Input: part model. Units: mm. Frame: model coordinates. Face numbers are marked on the shaded views. A direction names the side the tool comes from. Coordinates: 2 decimals unless noted, no trailing zeros. Order: outer loops, then holes, each group sorted by start corner. A loop starts at its lowest first (then second) coordinate and runs counter-clockwise, first axis right, second up. Notation, with made-up numbers: (22.5, 44) - (45.5, 44) arc R14 ccw to (45.5, 50) - close; hole circle Ø3 at (10.25, 6). An arc over 180 degrees is marked (long way). Answer as CSV lines item,"result". Start each with the question number.
Item 1: Material intervals for line 1 along Y through (x, z) = (-15, 31.4); line 2 along X through (y, z) = (-12.5, 31.6); line 3 along Z through (x, y) = (48.5, -15.5), sorted ascending.
Item 2: First-contact query: pin 1 (0.6 mm diameter, centred on x = -15, z = 29, fed in from +Y); pin 2 (4 mm diameter, centred on x = 20.5, z = 23.5, fed in from +Y); pin 3 (6.5 mm diameter, centred on x = -15, y = -0.5, fed in from -Z). Flat tips, straight axial feed; report the tip coordinate or a pass-through.
Item 3: Section C-C (z = 24.25). Output: boundary loops of the cut face in (x, y).
Item 4: Access query for the marked faces 1, 2 and 3. Directions: +Z, -Z, +X, -X, +Y, -Y. A direction counts if a zero-diameter tool reaches every point of the face in a straight line with its end or side. Return the directions, or none.
Item 5: Section B-B (x = -15). Output: boundary loops of the cut face in (y, z), and give its area (3 significant figures).
Item 6: Section A-A (y = 15.5). Output: boundary loops of the cut face in (x, z), and give its area (4 significant figures).
Item 7: Draft query along X for the marked faces 4, 5 and 6. Return one class per face: +X half, -X half, draft (parallel to the pull), parting line (faces both ways), or undercut.
Item 8: Section D-D (x = 13). Output: boundary loops of the cut face in (y, z).
from build123d import *

# Parameters (mm, degrees)
CYLINDER026_R     = 3.15
CYLINDER026_DEPTH = 10
CYLINDER027_R     = 3.15
CYLINDER027_DEPTH = 10
CYLINDER028_R     = 1.65
CYLINDER028_DEPTH = 83
CYLINDER029_R     = 1.65
CYLINDER029_DEPTH = 83
BOX022_W          = 50.5
BOX022_H          = 8
BOX022_DEPTH      = 9
CHAMFER026_SIZE   = 7
CYLINDER025_R     = 17
CYLINDER025_DEPTH = 83
BOX021_W          = 5
BOX021_H          = 57
BOX021_DEPTH      = 10
CHAMFER027_SIZE   = 1
BOX024_W          = 8
BOX024_H          = 16
BOX024_DEPTH      = 2
BOX036_W          = 28
BOX036_H          = 14
BOX036_DEPTH      = 10
BOX023_W          = 77.5
BOX023_H          = 57
BOX023_DEPTH      = 5
FILLET002_R       = 3


with BuildPart() as cylinder012:
    # Cylinder026 → Cylinder026 (new body)
    with BuildSketch(Plane(origin=(-15, 11.5, 26), x_dir=(1, 0, 0), z_dir=(0, 0, 1))):
        Circle(CYLINDER026_R)
    extrude(amount=CYLINDER026_DEPTH)


with BuildPart() as fusion006002011004053036004001028003008:
    # Cylinder027 → Cylinder027 (new body)
    with BuildSketch(Plane(origin=(-15, -12.5, 26), x_dir=(1, 0, 0), z_dir=(0, 0, 1))):
        Circle(CYLINDER027_R)
    extrude(amount=CYLINDER027_DEPTH)

    # Fusion006002011004053036004001028003008: union Cylinder012
    add(cylinder012.part)


with BuildPart() as obj1:
    # Cylinder028 → Cylinder028 (new body)
    with BuildSketch(Plane(origin=(25.5, -15.5, 24), x_dir=(0, 0, -1), z_dir=(1, 0, 0))):
        Circle(CYLINDER028_R)
    extrude(amount=CYLINDER028_DEPTH)


with BuildPart() as fusion006002011004053036004001024:
    # Cylinder029 → Cylinder029 (new body)
    with BuildSketch(Plane(origin=(25.5, 15.5, 24), x_dir=(0, 0, -1), z_dir=(1, 0, 0))):
        Circle(CYLINDER029_R)
    extrude(amount=CYLINDER029_DEPTH)

    # Fusion006002011004053036004001024: union obj1
    add(obj1.part)


with BuildPart() as chamfer026:
    # Box022 → Box022 (new body)
    with BuildSketch(Plane(origin=(0, -26.5, 22), x_dir=(1, 0, 0), z_dir=(0, 0, 1))):
        with Locations((25.25, 4)):
            Rectangle(BOX022_W, BOX022_H)
    extrude(amount=BOX022_DEPTH)

    # Chamfer026
    chamfer026_edges = [chamfer026.edges().sort_by_distance(p)[0] for p in [
        (25.25, -18.5, 22),
    ]]
    chamfer(chamfer026_edges, length=CHAMFER026_SIZE)


with BuildPart() as obj2:
    # Cylinder025 → Cylinder025 (new body)
    with BuildSketch(Plane(origin=(18.5, 0, 8.5), x_dir=(0, 0, -1), z_dir=(1, 0, 0))):
        Circle(CYLINDER025_R)
    extrude(amount=CYLINDER025_DEPTH)


with BuildPart() as cut001022:
    # Box021 → Box021 (new body)
    with BuildSketch(Plane(origin=(45.5, -26.5, 20.5), x_dir=(1, 0, 0), z_dir=(0, 0, 1))):
        with Locations((2.5, 28.5)):
            Rectangle(BOX021_W, BOX021_H)
    extrude(amount=BOX021_DEPTH)

    # Chamfer027
    chamfer027_edges = [cut001022.edges().sort_by_distance(p)[0] for p in [
        (48, -26.5, 20.5),
        (48, 30.5, 20.5),
    ]]
    chamfer(chamfer027_edges, length=CHAMFER027_SIZE)

    # Cut001022: cut obj2
    add(obj2.part, mode=Mode.SUBTRACT)


with BuildPart() as cube024:
    # Box024 → Box024 (new body)
    with BuildSketch(Plane(origin=(-19, -8.5, 28), x_dir=(1, 0, 0), z_dir=(0, 0, 1))):
        with Locations((4, 8)):
            Rectangle(BOX024_W, BOX024_H)
    extrude(amount=BOX024_DEPTH)


with BuildPart() as cube036:
    # Box036 → Box036 (new body)
    with BuildSketch(Plane(origin=(-30, 25.5, 25), x_dir=(1, 0, 0), z_dir=(0, 0, 1))):
        with Locations((14, 7)):
            Rectangle(BOX036_W, BOX036_H)
    extrude(amount=BOX036_DEPTH)


with BuildPart() as cut001024014:
    # Box023 → Box023 (new body)
    with BuildSketch(Plane(origin=(-27, -26.5, 30), x_dir=(1, 0, 0), z_dir=(0, 0, 1))):
        with Locations((38.75, 28.5)):
            Rectangle(BOX023_W, BOX023_H)
    extrude(amount=BOX023_DEPTH)

    # Cut001024012: cut Cube036
    add(cube036.part, mode=Mode.SUBTRACT)

    # Fillet002
    fillet002_edges = [cut001024014.edges().sort_by_distance(p)[0] for p in [
        (-27, 25.5, 32.5),
        (-27, -26.5, 32.5),
        (-2, 30.5, 32.5),
    ]]
    fillet(fillet002_edges, radius=FILLET002_R)

    # Fusion006002011004053036004001028003007: union Chamfer026, Cut001022, Cube024
    add(chamfer026.part)
    add(cut001022.part)
    add(cube024.part)

    # Cut001024013: cut Fusion006002011004053036004001024
    add(fusion006002011004053036004001024.part, mode=Mode.SUBTRACT)

    # Cut001024014: cut Fusion006002011004053036004001028003008
    add(fusion006002011004053036004001028003008.part, mode=Mode.SUBTRACT)


solid = cut001024014.part
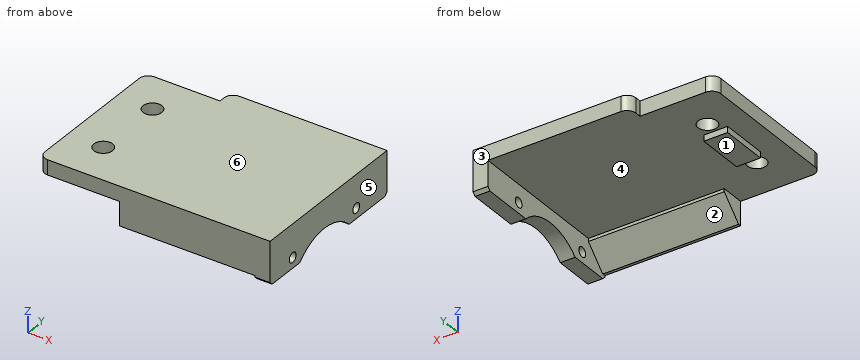
Determined:
1,line 1,"y = -26.5 to -15.65, -9.35 to 8.35, 14.65 to 25.5"
1,line 2,"x = -27 to -18.15, -11.85 to 50.5"
1,line 3,"z = 20.5 to 22.35, 25.65 to 35"
2,pin 1,"stops at y = 7.5"
2,pin 2,"stops at y = -22"
2,pin 3,"stops at z = 28"
3,outline,"(0, -26.5) - (50.5, -26.5) - (50.5, -17.13) - (45.5, -17.13) - (45.5, -23.25) - (0, -23.25) - close; (45.5, -13.87) - (50.5, -13.87) - (50.5, -6.4) - (45.5, -6.4) - close; (45.5, 6.4) - (50.5, 6.4) - (50.5, 13.87) - (45.5, 13.87) - close; (45.5, 17.13) - (50.5, 17.13) - (50.5, 30.5) - (45.5, 30.5) - close"
4,face 1,"-Z, -X, +Y, -Y"
4,face 2,"-Z, -X, +Y"
4,face 3,"+Z, -Z, +X, -X, +Y"
5,outline,"(-26.5, 30) - (-15.65, 30) - (-15.65, 35) - (-26.5, 35) - close; (-9.35, 30) - (-8.5, 30) - (-8.5, 28) - (7.5, 28) - (7.5, 30) - (8.35, 30) - (8.35, 35) - (-9.35, 35) - close; (14.65, 30) - (25.5, 30) - (25.5, 35) - (14.65, 35) - close"
5,area,"229 mm^2"
6,outline,"(-27, 30) - (45.5, 30) - (45.5, 25.65) - (50.5, 25.65) - (50.5, 35) - (-27, 35) - close; (45.5, 20.5) - (50.5, 20.5) - (50.5, 22.35) - (45.5, 22.35) - close"
6,area,"418.5 mm^2"
7,face 4,"undercut"
7,face 5,"+X half"
7,face 6,"draft"
8,outline,"(-26.5, 22) - (-25.5, 22) - (-18.5, 29) - (-18.5, 30) - (30.5, 30) - (30.5, 35) - (-26.5, 35) - close"
